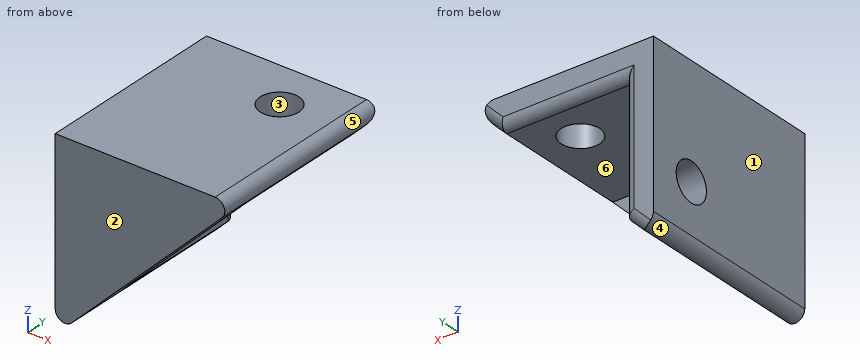
```python
from build123d import *

# Parameters (mm, degrees)
BOSS_EXTRUDE1_DEPTH = 5
BOSS_EXTRUDE2_DEPTH = 15
SKETCH3_R           = 2
CUT_EXTRUDE1_DEPTH  = 34.496268449
SKETCH4_R           = 2
CUT_EXTRUDE2_DEPTH  = 34.496268449
FILLET1_R           = 1


with BuildPart() as part:
    # Sketch1 → Boss-Extrude1 (new body)
    with BuildSketch(Plane(origin=(0, 0, 0), x_dir=(1, 0, 0), z_dir=(0, 1, 0))):
        Polygon((0, 0), (0, 19), (19, 0), align=None)
    extrude(amount=BOSS_EXTRUDE1_DEPTH)

    # Sketch2 → Boss-Extrude2 (add)
    with BuildSketch(Plane(origin=(0, 5, 0), x_dir=(1, 0, 0), z_dir=(0, 1, 0))):
        Polygon((0, 19), (0, 0), (19, 0), (16, 3), (3, 3), (3, 16), align=None)
    extrude(amount=BOSS_EXTRUDE2_DEPTH)

    # Sketch3 → Cut-Extrude1 (cut, through all)
    with BuildSketch(Plane.XY):
        with Locations((11.5, 15)):
            Circle(SKETCH3_R)
    extrude(amount=-CUT_EXTRUDE1_DEPTH, mode=Mode.SUBTRACT)

    # Sketch4 → Cut-Extrude2 (cut, through all)
    with BuildSketch(Plane.ZY):
        with Locations((-11.5, 15)):
            Circle(SKETCH4_R)
    extrude(amount=-CUT_EXTRUDE2_DEPTH, mode=Mode.SUBTRACT)

    # Fillet1
    fillet1_edges = [part.edges().sort_by_distance(p)[0] for p in [
        (9.5, 20, -3),
        (3, 20, -9.5),
        (1.5, 20, -17.5),
        (17.5, 20, -1.5),
        (19, 10, 0),
        (0, 10, -19),
    ]]
    fillet(fillet1_edges, radius=FILLET1_R)


solid = part.part
```
Geometry: final body of the model. Coordinates: model frame, mm. Face numbers are marked on the shaded views. A direction names the side the tool comes from. Round coordinates to 2 decimals unless told otherwise and drop trailing zeros. Order: outer loops, then holes, each group sorted by start corner. A loop starts at its lowest first (then second) coordinate and runs counter-clockwise, first axis right, second up. Notation, with made-up numbers: M 73,61 L 118,61 A23 ccw 118,96 Z; hole C 78,-14.75 d8. An arc over 180 degrees is marked long. Use one line per item in the form item = value. Start each with the question number.
Q1. Cut plane B-B (z = -11.5). Return loops of the section in (x, y), and give its area (3 significant figures).
Q2. Material intervals for line 1 (Y direction, x = 11.5, z = -1.95); line 2 (X direction, y = 6, z = -9); line 3 (Z direction, x = 4.5, y = 15.5), sorted ascending. Write a range as [from, to].
Q3. Pin query (flat end, axial travel): pin 1 Ø4 at (x, y) = (6, 3.5) entering from -Z; pin 2 Ø3 at (x, z) = (9.5, -11.5) entering from +Y; pin 3 Ø10.5 at (y, z) = (13, -10) entering from +X. Return the tip coordinate at first contact, or that it passes through.
Q4. Cut plane A-A (x = 11.5). Return loops of the section in (y, z).
Q5. Cut plane D-D (x = 14.75). Return loops of the section in (y, z).
Q6. Access query for the marked faces 5 and 6. Directions: +Z, -Z, +X, -X, +Y, -Y. A direction counts if a zero-diameter tool reaches every point of the face in a straight line with its end or side. Return the directions, or none.
Q7. Cut plane C-C (y = 15). Return loops of the section in (x, z), and give its area (3 significant figures).
Q8. Mould query, pull axis X, two halves, no side actions, for the marked faces 1, 2, 3 and 4. Classes: +X half, -X half, draft (parallel to the pull), parting line (faces both ways), or undercut.
Geometry results:
q1.outline = M 0,0 L 7.5,0 L 7.5,5 L 3,5 L 3,13 L 0,13 Z; M 0,17 L 3,17 L 3,19 A1 ccw 2,20 L 0,20 Z
q1.area = 70.3 mm^2
q2.line_1 = [0, 13], [17, 20]
q2.line_2 = [0, 3]
q2.line_3 = [-3, 0]
q3.pin_1 = -15
q3.pin_2 = 5
q3.pin_3 = 3
q4.outline = M 0,-7.5 L 5,-7.5 L 5,-3 L 13,-3 L 13,0 L 0,0 Z; M 17,-3 L 19,-3 A1 ccw 20,-2 L 20,0 L 17,0 Z
q5.outline = M 0,-4.25 L 5,-4.25 L 5,-3 L 19,-3 A1 ccw 20,-2 L 20,0 L 0,0 Z
q6.face_5 = +X, +Y, -Y
q6.face_6 = -Z, +X, +Y
q7.outline = M 0,-16.59 A1 ccw 1.71,-17.29 L 3,-16 L 3,-13.5 L 0,-13.5 Z; M 0,-9.5 L 3,-9.5 L 3,-3 L 9.5,-3 L 9.5,0 L 0,0 Z; M 13.5,-3 L 16,-3 L 17.29,-1.71 A1 ccw 16.59,0 L 13.5,0 Z
q7.area = 69.5 mm^2
q8.face_1 = -X half
q8.face_2 = draft
q8.face_3 = undercut
q8.face_4 = parting line
